CAD build for the part. Positions are in the model's coordinates, mm. A direction names the side the tool comes from. Give positions to 0.01 mm unless a question says otherwise; leave off trailing zeros. Write each loop counter-clockwise with the first axis right and the second up, starting at its lowest first coordinate (ties: lowest second). Pieces come first, ordered by that corner, then holes. Notation, with made-up numbers: (73.25, 79.5) -> (107.25, 79.5) arc R36 cw to (107.25, 116.5) -> close; hole circle Ø2 at (39, -23.75). An arc over 180 degrees is marked (long way). Use one line per item in the form item = value. Start each with the question number.
from build123d import *

# Parameters (mm, degrees)
F2_DEPTH = 5.5
F3_R     = 5
F4_D     = 16.15
F5_R     = 1.5


with BuildPart() as f2:
    # F1 (on Top) → F2 (new body)
    with BuildSketch(Plane.XY):
        with BuildLine():
            ThreePointArc((-26.6506350946, 3.8397459622), (-16.6506350946, 3.8397459622), (-11.6506350946, 12.5))
            ThreePointArc((-11.6506350946, 12.5), (-12.9903810568, 17.5), (-16.6506350946, 21.1602540378))
            ThreePointArc((-16.6506350946, 21.1602540378), (-30.3108891325, 17.5), (-26.6506350946, 3.8397459622))
        make_face()
        with BuildLine():
            ThreePointArc((-16.6506350946, 21.1602540378), (-12.9903810568, 17.5), (-11.6506350946, 12.5))
            ThreePointArc((-11.6506350946, 12.5), (-16.6506350946, 3.8397459622), (-26.6506350946, 3.8397459622))
            Line((-26.6506350946, 3.8397459622), (-10, -5.7735026919))
            Line((-10, -5.7735026919), (-10, -25))
            ThreePointArc((-10, -25), (0, -15), (10, -25))
            Line((10, -25), (10, -5.7735026919))
            Line((10, -5.7735026919), (26.6506350946, 3.8397459622))
            ThreePointArc((26.6506350946, 3.8397459622), (12.9903810568, 7.5), (16.6506350946, 21.1602540378))
            Line((16.6506350946, 21.1602540378), (0, 11.5470053838))
            Line((0, 11.5470053838), (-16.6506350946, 21.1602540378))
        make_face()
        with BuildLine():
            ThreePointArc((31.6506350946, 12.5), (26.6506350946, 21.1602540378), (16.6506350946, 21.1602540378))
            ThreePointArc((16.6506350946, 21.1602540378), (12.9903810568, 7.5), (26.6506350946, 3.8397459622))
            ThreePointArc((26.6506350946, 3.8397459622), (30.3108891325, 7.5), (31.6506350946, 12.5))
        make_face()
        with BuildLine():
            ThreePointArc((10, -25), (0, -15), (-10, -25))
            ThreePointArc((-10, -25), (0, -35), (10, -25))
        make_face()
    extrude(amount=F2_DEPTH)

    # F3
    f3_edges = [f2.edges().sort_by_distance(p)[0] for p in [
        (-10, -5.773503, 2.75),
        (10, -5.773503, 2.75),
        (0, 11.547005, 2.75),
    ]]
    fillet(f3_edges, radius=F3_R)

    # F4 (through all)
    with Locations(Plane(origin=(0, 0, 0), x_dir=(1, 0, 0), z_dir=(0, 0, -1))):
        with Locations((0, 25), (-21.6506350946, -12.5), (21.6506350946, -12.5), (0, 0)):
            Hole(F4_D / 2)

    # F5
    f5_edges = [f2.edges().sort_by_distance(p)[0] for p in [
        (-19.575318, -0.245191, 5.5),
        (-10, -16.830127, 0),
    ]]
    fillet(f5_edges, radius=F5_R)


solid = f2.part
1) Cut at C-C (y = -13). Give the cut face in (x, z).
2) Wall check: line 1 along Y through (x, z) = (0, 2.15) (1 decimal); line 2 along X through (y, z) = (10.5, 2.4); line 3 along Y through (x, z) = (-3, 1.2). Give the ranges that are in metal, low to high. Write a range as from..to.
3) Cut at D-D (y = -19). Give the cut face in (x, z), and give its area (3 significant figures).
4) Cut at A-A (x = 0). Give the cut face in (y, z) (1 decimal).
5) Cut at B-B (z = 2.8). State how many separate pieces and enclosed holes the cut face has, and give its area (3 significant figures).
6) Two-plate mould, pull along Y, no slides. Class faces 1 (the face through (17.92, 19.66, 2.79)), 2 (the face through (-9.48, 17.02, 2.73)), 3 (the face through (-19.251, 0.088, 0.428)): released by +Y, released by -Y, zero draft, split by the parting line, or undercut.
7) 3-axis set-ups, long thin cutter, end or side, ignore diameter. For faces 4 (the face through (10, -17, 3)), 5 (the face through (9.7, 16.63, 0.43)), 6 (the face through (9.69, 16.648, 5.049)): which of +Z, -Z, +X, -X, +Y, -Y reach the whole face in a straight line?
8) Pin check, flat tips, straight feed: pin 1 (1 mm diameter, centred on y = -11.5, z = 1, fed in from -X); pin 2 (18.5 mm diameter, centred on x = 21.65, y = 12.5, fed in from +Z); pin 3 (3 mm diameter, centred on x = -3.5, z = 5, fed in from -Y); pin 4 (2 mm diameter, centred on y = -16.5, z = 2.5, fed in from +X). Stop position of each tip, or through.
Final values:
q1.outline = (-10, 1.5) arc R1.5 ccw to (-8.5, 0) -> (8.5, 0) arc R1.5 ccw to (10, 1.5) -> (10, 4) arc R1.5 ccw to (8.5, 5.5) -> (-8.5, 5.5) arc R1.5 ccw to (-10, 4) -> close
q2.line_1 = -35..-33.1, -16.9..-8.1, 8.1..12.3
q2.line_2 = -31.45..-29.47, -13.83..13.83, 29.47..31.45
q2.line_3 = -34.51..-32.5, -17.5..-7.5, 7.5..13.24
q3.outline = (-10, 1.5) arc R1.5 ccw to (-8.5, 0) -> (-5.4, 0) -> (-5.4, 5.5) -> (-8.5, 5.5) arc R1.5 ccw to (-10, 4) -> close; (5.4, 0) -> (8.5, 0) arc R1.5 ccw to (10, 1.5) -> (10, 4) arc R1.5 ccw to (8.5, 5.5) -> (5.4, 5.5) -> close
q3.area = 48.6 mm^2
q4.outline = (-35, 1.5) arc R1.5 ccw to (-33.5, 0) -> (-33.1, 0) -> (-33.1, 5.5) -> (-33.5, 5.5) arc R1.5 ccw to (-35, 4) -> close; (-16.9, 0) -> (-8.1, 0) -> (-8.1, 5.5) -> (-16.9, 5.5) -> close; (8.1, 0) -> (10.8, 0) arc R1.5 ccw to (12.3, 1.5) -> (12.3, 4) arc R1.5 ccw to (10.8, 5.5) -> (8.1, 5.5) -> close
q5.separate_pieces = 1
q5.enclosed_holes = 4
q5.area = 983 mm^2
q6.face_1 = undercut
q6.face_2 = released by +Y
q6.face_3 = released by -Y
q7.face_4 = +Z, -Z, +X, -Y
q7.face_5 = -Z, +Y
q7.face_6 = +Z, +Y
q8.pin_1 = -10
q8.pin_2 = 5.5
q8.pin_3 = -34.73
q8.pin_4 = 10
